Verification items for this drawing (mm, ordinates from the low corner). A direction names the side the tool comes from. Give positions to 0.01 mm unless a question says otherwise; leave off trailing zeros. Write each loop counter-clockwise with the first axis right and the second up, starting at its lowest first coordinate (ties: lowest second). Pieces come first, ordered by that corner, then holes. Notation, with made-up numbers: (49.5, 53.5) -> (74.5, 53.5) arc R25 cw to (74.5, 65.5) -> close; hole circle Ø2 at (31.25, 60.5). An arc over 180 degrees is marked (long way). One line per item, written item: value.
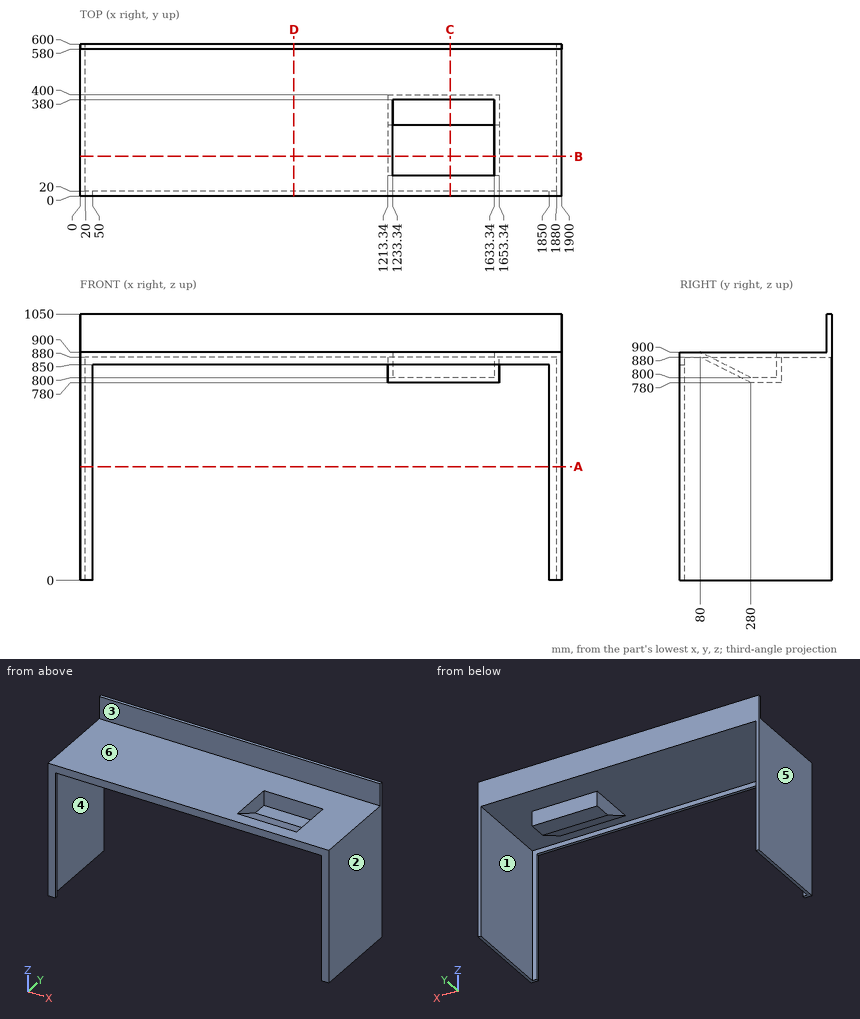
1) Depth check by flat-ended pin: pin 1 Ø5 at (x, y) = (1196.5, 274) entering from +Z; pin 2 Ø10 at (x, y) = (1052, 313.5) entering from -Z; pin 3 Ø1.5 at (y, z) = (485.5, 607.5) entering from -X; pin 4 Ø6 at (x, y) = (1232.5, 8.5) entering from -Z. Enter the tip coordinate at first touch or a pass-through.
Verdict:
pin 1: z = 900
pin 2: z = 880
pin 3: x = 0
pin 4: z = 850
2) Mould release check, pull along X, two halves, no side actions. Record for the marked faces 1, 2 and 3: released by +X, released by -X, zero draft, split by the parting line, or undercut.
Verdict:
face 1: undercut
face 2: released by +X
face 3: zero draft
3) Sectioned sample at C-C on x = 1459.5. Record the cut outline in (y, z), plus the area to 3 significant figures.
Verdict:
outline: (0, 850) -> (20, 850) -> (20, 880) -> (80, 880) -> (280, 780) -> (400, 780) -> (400, 880) -> (600, 880) -> (600, 1050) -> (580, 1050) -> (580, 900) -> (380, 900) -> (380, 800) -> (280, 800) -> (80, 900) -> (0, 900) -> close
area: 17,600 mm^2
4) Scan lines: probe 1 along X at (y, z) = (494, 334); probe 2 along Y at (x, z) = (1468, 854); probe 3 along Z at (x, y) = (259.5, 507.5). Record each from-to range of solid material in increasing order.
Verdict:
probe 1: 0 to 20, 1880 to 1900
probe 2: 0 to 20, 132 to 172, 380 to 400
probe 3: 880 to 900
5) Tool access check on the marked faces 4, 5 and 6. Record the directions out of +Z, -Z, +X, -X, +Y, -Y that give a thin tool (end or side, any length) a straight path to the whole face; none if there is none.
Verdict:
face 4: -Z, +Y
face 5: +Z, -Z, -X, +Y, -Y
face 6: +Z, +X, -X, -Y
6) Sectioned sample at A-A on z = 449. Record the cut outline in (x, y).
Verdict:
outline: (0, 0) -> (50, 0) -> (50, 20) -> (20, 20) -> (20, 600) -> (0, 600) -> close; (1850, 0) -> (1900, 0) -> (1900, 600) -> (1880, 600) -> (1880, 20) -> (1850, 20) -> close
7) Sectioned sample at D-D on x = 843. Record the cut outline in (y, z).
Verdict:
outline: (0, 850) -> (20, 850) -> (20, 880) -> (600, 880) -> (600, 1050) -> (580, 1050) -> (580, 900) -> (0, 900) -> close
8) Sectioned sample at B-B on y = 157. Record the cut outline in (x, z).
Verdict:
outline: (0, 0) -> (20, 0) -> (20, 880) -> (1213.34, 880) -> (1213.34, 841.5) -> (1653.34, 841.5) -> (1653.34, 880) -> (1880, 880) -> (1880, 0) -> (1900, 0) -> (1900, 900) -> (1633.34, 900) -> (1633.34, 861.5) -> (1233.34, 861.5) -> (1233.34, 900) -> (0, 900) -> close
